from build123d import *

# Parameters (mm, degrees)
F0_W = 1.905
F0_H = 0.254


# Not quite as in the source:
# - a fillet or chamfer that OpenCascade refuses, or shapes differently, is made with other operations: its cross-section is extruded or revolved along the edge and cut away or added


with BuildPart() as f1:
    # F0 (on Front) → F1 (revolve)
    with BuildSketch(Plane.XZ):
        with Locations((-29.5277546042, 20.4458203979)):
            Rectangle(F0_W, F0_H)
        Polygon((-30.4802546042, 20.3188203979), (-30.4802546042, 20.5728203979), (-32.1947546042, 20.5728203979), (-32.1947546042, 12.6988203979), (-30.4802546042, 12.6988203979), (-30.4802546042, 12.9528203979), align=None)
        with Locations((-29.5277546042, 12.8258203979)):
            Rectangle(F0_W, F0_H)
    revolve(axis=Axis((-32.1947546042, 0, 16.6358203979), (0, 0, 1)))

    # F2: fillet of radius 2.286 on 1 edges, made by hand

    # F2_s1 → F2_t2 (revolve, cut)
    with BuildSketch(Plane.XZ):
        with BuildLine():
            ThreePointArc((-29.6225234331, 20.5728203979), (-29.0837080659, 20.5084130698), (-28.5752546042, 20.3188203979))
            Line((-28.5752546042, 20.3188203979), (-28.5752546042, 20.5728203979))
            Line((-28.5752546042, 20.5728203979), (-29.6225234331, 20.5728203979))
        make_face()
    revolve(axis=Axis((-32.1947546042, 0, 20.5728203979), (0, 0, 1)), mode=Mode.SUBTRACT)

    # F3: fillet of radius 2.286 on 1 edges, made by hand

    # F3_s1 → F3_t2 (revolve, cut)
    with BuildSketch(Plane.XZ):
        with BuildLine():
            ThreePointArc((-28.5752546042, 12.9528203979), (-29.0837080659, 12.763227726), (-29.6225234331, 12.6988203979))
            Line((-29.6225234331, 12.6988203979), (-28.5752546042, 12.6988203979))
            Line((-28.5752546042, 12.6988203979), (-28.5752546042, 12.9528203979))
        make_face()
    revolve(axis=Axis((-32.1947546042, 0, 12.6988203979), (0, 0, 1)), mode=Mode.SUBTRACT)


solid = f1.part
Could you check a few things on this model? Use its own coordinates, in mm. Coordinates: 2 decimals unless noted, no trailing zeros. Order: outer loops, then holes, each group sorted by start corner. A loop starts at its lowest first (then second) coordinate and runs counter-clockwise, first axis right, second up.
Q1. Thinking about a two-plate mould opening in Z: for faces 1 (the flat face through (-32, 0, 20.573)), 2 (the flat face through (-34, -1, 12.953)), 3 (the flat face through (-34, -1, 20.319)), 4 (the flat face through (-32, 0, 12.699)), which applies, released by +Z, released by -Z, zero draft, split by the parting line, or undercut?
Q2. Please list where these lines run through material, in increasing order: L1, parallel to Z at x = -30, y = 0.5; L2, parallel to Y at x = -32.25, z = 15.25; L3, parallel to Z at x = -32, y = 3.
Q3. Suppose I cut it at A-A on y = 0. Please give me the cut outline in (x, z), and give its area (3 significant figures).
Q4. Will these pins go through, and if not, where does the flat tip stop? pin 1 (2 mm diameter, centred on y = -2.5, z = 15.5, fed in from +X); pin 2 (1.5 mm diameter, centred on x = -31.5, z = 18, fed in from -Y); pin 3 (4 mm diameter, centred on x = -34, z = 18, fed in from +Y).
Q5. Suppose I cut it at B-B on z = 15.25. Please give me the cut outline in (x, y), and give its area (3 significant figures).
Answer:
1. face 1: released by +Z
1. face 2: undercut
1. face 3: undercut
1. face 4: released by -Z
2. L1: z = 12.7 to 12.95, 20.32 to 20.57
2. L2: y = -1.71 to 1.71
2. L3: z = 12.74 to 12.95, 20.32 to 20.53
3. outline: (-35.81, 12.95) arc R2.29 ccw to (-34.77, 12.7) - (-29.62, 12.7) arc R2.29 ccw to (-28.58, 12.95) - (-30.48, 12.95) - (-30.48, 20.32) - (-28.58, 20.32) arc R2.29 ccw to (-29.62, 20.57) - (-34.77, 20.57) arc R2.29 ccw to (-35.81, 20.32) - (-33.91, 20.32) - (-33.91, 12.95) - close
3. area: 28.6 mm2
4. pin 1: stops at x = -31.36
4. pin 2: stops at y = -1.71
4. pin 3: stops at y = 1.71
5. outline: circle Ø3.43 at (-32.19, 0)
5. area: 9.23 mm2
